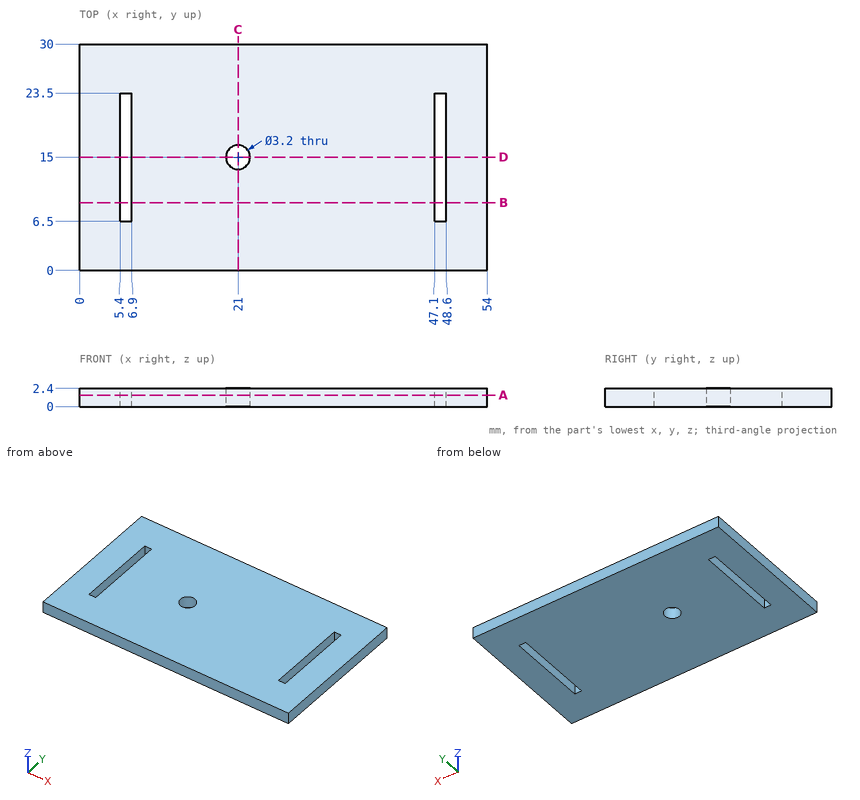
Print and shaded views of the part. All mm, measured from the part's lowest x, y and z. Round coordinates to 2 decimals unless told otherwise and drop trailing zeros. Write each loop counter-clockwise with the first axis right and the second up, starting at its lowest first coordinate (ties: lowest second). Pieces come first, ordered by that corner, then holes. Notation, with made-up numbers: (11, 37.5) -> (32, 37.5) arc R20 cw to (32, 54.5) -> close; hole circle Ø8 at (63.25, 40.5). An arc over 180 degrees is marked (long way). Answer in a Markdown table with one row per item. Add a question column.
Item 1: Drill centre lines: line 1 (X direction, y = 22.25, z = 0.2); line 2 (Y direction, x = 21, z = 0.8); line 3 (X direction, y = 15.75, z = 0.1). Where is each one in solid material? Low to high. Write a range as from..to.
Item 2: Saw through at A-A, the plane z = 1.5. Write the cut outline in (x, y).
Item 3: Drop a flat-ended pin along its axis: pin 1 Ø2.5 at (x, y) = (21, 15) entering from -Z. Give the stop position or say it passes through.
Item 4: Saw through at C-C, the plane x = 21. Write the cut outline in (y, z).
Item 5: Saw through at D-D, the plane y = 15. Write the cut outline in (x, z), then the cut area to 3 significant figures.
Item 6: Saw through at B-B, the plane y = 9. Write the cut outline in (x, z).
Findings below:
| question | item | result |
|---|---|---|
| 1 | line 1 | x = 0..5.4, 6.9..47.1, 48.6..54 |
| 1 | line 2 | y = 0..13.4, 16.6..30 |
| 1 | line 3 | x = 0..5.4, 6.9..19.59, 22.41..47.1, 48.6..54 |
| 2 | outline | (0, 0) -> (54, 0) -> (54, 30) -> (0, 30) -> close; hole (5.4, 6.5) -> (6.9, 6.5) -> (6.9, 23.5) -> (5.4, 23.5) -> close; hole circle Ø3.2 at (21, 15); hole (47.1, 6.5) -> (48.6, 6.5) -> (48.6, 23.5) -> (47.1, 23.5) -> close |
| 3 | pin 1 | passes through |
| 4 | outline | (0, 0) -> (13.4, 0) -> (13.4, 2.4) -> (0, 2.4) -> close; (16.6, 0) -> (30, 0) -> (30, 2.4) -> (16.6, 2.4) -> close |
| 5 | outline | (0, 0) -> (5.4, 0) -> (5.4, 2.4) -> (0, 2.4) -> close; (6.9, 0) -> (19.4, 0) -> (19.4, 2.4) -> (6.9, 2.4) -> close; (22.6, 0) -> (47.1, 0) -> (47.1, 2.4) -> (22.6, 2.4) -> close; (48.6, 0) -> (54, 0) -> (54, 2.4) -> (48.6, 2.4) -> close |
| 5 | area | 115 mm^2 |
| 6 | outline | (0, 0) -> (5.4, 0) -> (5.4, 2.4) -> (0, 2.4) -> close; (6.9, 0) -> (47.1, 0) -> (47.1, 2.4) -> (6.9, 2.4) -> close; (48.6, 0) -> (54, 0) -> (54, 2.4) -> (48.6, 2.4) -> close |
